```python
from build123d import *

# Parameters (mm, degrees)
F0_W     = 17.4
F0_H     = 15.4
F1_DEPTH = 14
F2_W     = 15
F2_H     = 13
F3_DEPTH = 12
F4_W     = 4
F4_H     = 4
F5_DEPTH = 1.2


with BuildPart() as f1:
    # F0 (on Top) → F1 (new body)
    with BuildSketch(Plane.XY):
        Rectangle(F0_W, F0_H)
    extrude(amount=F1_DEPTH)

    # F2 (on face) → F3 (cut)
    with BuildSketch(Plane.XY.offset(14)):
        Rectangle(F2_W, F2_H)
    extrude(amount=-F3_DEPTH, mode=Mode.SUBTRACT)

    # F4 (on face) → F5 (cut)
    with BuildSketch(Plane.XZ.offset(-6.5)):
        with Locations((-5.5, 4)):
            Rectangle(F4_W, F4_H)
    extrude(amount=-F5_DEPTH, mode=Mode.SUBTRACT)


solid = f1.part
```
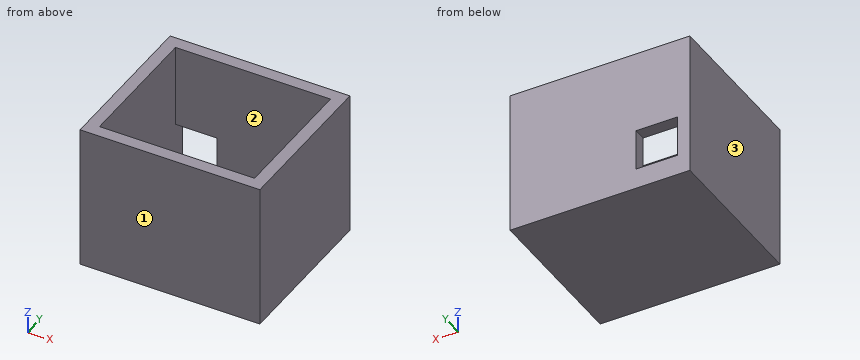
Read the model definition and answer for the solid it produces. Units are mm, in the model's axes. Face numbers are marked on the shaded views. Coordinates: 2 decimals unless noted, no trailing zeros. Write each loop counter-clockwise with the first axis right and the second up, starting at its lowest first coordinate (ties: lowest second). Pieces come first, ordered by that corner, then holes. Notation, with made-up numbers: (-16.5, -31.5) -> (25.5, -31.5) arc R19 ccw to (25.5, 4.5) -> close; hole circle Ø5 at (-19.5, -27). An arc over 180 degrees is marked (long way). Answer as a JSON object with one key per item and string values.
Q1. The part is cut by section C-C on z = 4.5. Give the vertices of the cut face in (x, y).
The answers:
{"outline": "(-8.7, -7.7) -> (8.7, -7.7) -> (8.7, 7.7) -> (-3.5, 7.7) -> (-3.5, 6.5) -> (7.5, 6.5) -> (7.5, -6.5) -> (-7.5, -6.5) -> (-7.5, 7.7) -> (-8.7, 7.7) -> close"}
Q2. Consider line 1 (X direction, y = -6.25, z = 7.25); line 2 (Y direction, x = 6, z = 4); line 3 (Z direction, x = 0.5, y = -1.25). Determine where each line is inside the solid, lowest interval first. Write a range as [from, to].
The answers:
{"line 1": "x = [-8.7, -7.5], [7.5, 8.7]", "line 2": "y = [-7.7, -6.5], [6.5, 7.7]", "line 3": "z = [0, 2]"}
Q3. The part is cut by section D-D on y = -1. Give the vertices of the cut face in (x, z), then the cut area to 3 significant figures.
The answers:
{"outline": "(-8.7, 0) -> (8.7, 0) -> (8.7, 14) -> (7.5, 14) -> (7.5, 2) -> (-7.5, 2) -> (-7.5, 14) -> (-8.7, 14) -> close", "area": "63.6 mm2"}
Q4. The part is cut by section A-A on x = -5. Give the vertices of the cut face in (y, z), then the cut area to 3 significant figures.
The answers:
{"outline": "(-7.7, 0) -> (7.7, 0) -> (7.7, 2) -> (-6.5, 2) -> (-6.5, 14) -> (-7.7, 14) -> close; (6.5, 6) -> (7.7, 6) -> (7.7, 14) -> (6.5, 14) -> close", "area": "54.8 mm2"}
Q5. The part is cut by section B-B on z = 6.25. Give the vertices of the cut face in (x, y).
The answers:
{"outline": "(-8.7, -7.7) -> (8.7, -7.7) -> (8.7, 7.7) -> (-8.7, 7.7) -> close; hole (-7.5, -6.5) -> (7.5, -6.5) -> (7.5, 6.5) -> (-7.5, 6.5) -> close"}
Q6. Flat-ended cylindrical pins translate along their axes: pin 1 Ø1 at (x, y) = (-6, 7) entering from -Z; pin 2 Ø7 at (x, y) = (-2.5, -2) entering from +Z. Find the tip coordinate at first contact, or state that the pin passes through.
The answers:
{"pin 1": "stops at z = 0", "pin 2": "stops at z = 2"}
Q7. Determine the mould class of the marked faces 1, 2 and 3 for opening direction Y: pulls with the +Y half, pulls with the -Y half, needs draft (parallel to the pull), parting line crosses it, or undercut.
The answers:
{"face 1": "pulls with the -Y half", "face 2": "undercut", "face 3": "needs draft"}
